Model file for the job. Use its own axes, mm. Face numbers are marked on the shaded views. A direction names the side the tool comes from. Give positions to 0.01 mm unless a question says otherwise; leave off trailing zeros. Loops run counter-clockwise (first coordinate to the right, second up) from the corner with the lowest first, then second, coordinate; pieces in that order, holes last. Notation, with made-up numbers: M -30,26 L -22,26 A9 cw -22,40 Z; hole C 32.25,44.25 d4. An arc over 180 degrees is marked long. Answer in a Markdown table with one row per item.
```python
from build123d import *

# Parameters (mm, degrees)
SKETCH1_W           = 25
SKETCH1_H           = 15.5
BOSS_EXTRUDE1_DEPTH = 15
SKETCH2_R           = 2.5
CUT_EXTRUDE1_DEPTH  = 10
SKETCH4_R           = 2.5
CUT_EXTRUDE3_DEPTH  = 4
SKETCH5_R           = 2.5
CUT_EXTRUDE4_DEPTH  = 4


with BuildPart() as part:
    # Sketch1 → Boss-Extrude1 (new body)
    with BuildSketch(Plane(origin=(0, 0, 0), x_dir=(1, 0, 0), z_dir=(0, 1, 0))):
        Rectangle(SKETCH1_W, SKETCH1_H)
    extrude(amount=BOSS_EXTRUDE1_DEPTH)

    # Sketch2 → Cut-Extrude1 (cut)
    with BuildSketch(Plane(origin=(0, 15, 0), x_dir=(1, 0, 0), z_dir=(0, 1, 0))):
        Circle(SKETCH2_R)
    extrude(amount=-CUT_EXTRUDE1_DEPTH, mode=Mode.SUBTRACT)

    # Sketch4 → Cut-Extrude3 (cut)
    with BuildSketch(Plane.XZ):
        with Locations((5, 0)):
            Circle(SKETCH4_R)
    extrude(amount=-CUT_EXTRUDE3_DEPTH, mode=Mode.SUBTRACT)

    # Sketch5 → Cut-Extrude4 (cut)
    with BuildSketch(Plane.XZ):
        with Locations((-5, 0)):
            Circle(SKETCH5_R)
    extrude(amount=-CUT_EXTRUDE4_DEPTH, mode=Mode.SUBTRACT)


solid = part.part
```
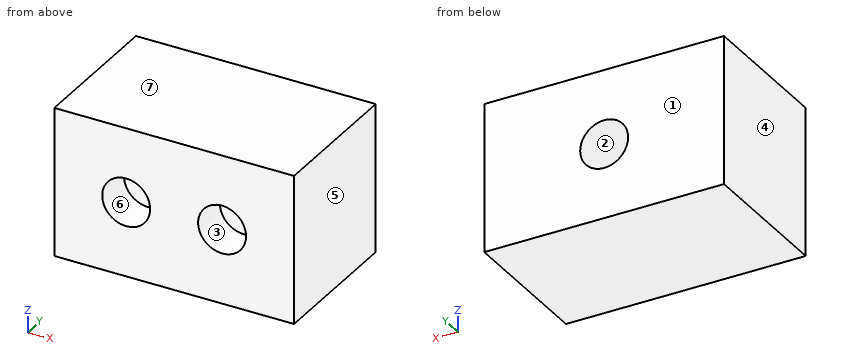
(1) Saw through at C-C, the plane y = 13.5. Give the cut face in (x, z).
Established:
| item | result |
|---|---|
| outline | M -12.5,-7.75 L 12.5,-7.75 L 12.5,7.75 L -12.5,7.75 Z; hole C 0,0 d5 |
(2) Saw through at B-B, the plane z = 0. Give the cut face in (x, y).
Established:
| item | result |
|---|---|
| outline | M -12.5,0 L -7.5,0 L -7.5,4 L -2.5,4 L -2.5,0 L 2.5,0 L 2.5,4 L 7.5,4 L 7.5,0 L 12.5,0 L 12.5,15 L 2.5,15 L 2.5,5 L -2.5,5 L -2.5,15 L -12.5,15 Z |
(3) Wall check: L1, parallel to Z at x = -5, y = 2.55; L2, parallel to X at y = 11.5, z = 0; L3, parallel to Y at x = 0, z = -0.5. Give the ranges that are in metal, low to high.
Established:
| item | result |
|---|---|
| L1 | z = -7.75 to -2.5, 2.5 to 7.75 |
| L2 | x = -12.5 to -2.5, 2.5 to 12.5 |
| L3 | y = 0 to 5 |
(4) Saw through at D-D, the plane x = -7. Give the cut face in (y, z).
Established:
| item | result |
|---|---|
| outline | M 0,-7.75 L 15,-7.75 L 15,7.75 L 0,7.75 L 0,1.5 L 4,1.5 L 4,-1.5 L 0,-1.5 Z |
(5) Which spindle directions (+Z, -Z, +X, -X, +Y, -Y) get a long thin tool onto all of the face, cutting with end or side? Do the marked faces 1, 2 and 3. Say none if no direction does.
Established:
| item | result |
|---|---|
| face 1 | +Z, -Z, +X, -X, +Y |
| face 2 | +Y |
| face 3 | -Y |
(6) Mould opens along X. For the marked faces 4, 5, 6 and 7 say: pulls with the +X half, pulls with the -X half, needs draft (parallel to the pull), parting line crosses it, or undercut.
Established:
| item | result |
|---|---|
| face 4 | pulls with the -X half |
| face 5 | pulls with the +X half |
| face 6 | undercut |
| face 7 | needs draft |
(7) Saw through at A-A, the plane x = 0. Give the cut face in (y, z).
Established:
| item | result |
|---|---|
| outline | M 0,-7.75 L 15,-7.75 L 15,-2.5 L 5,-2.5 L 5,2.5 L 15,2.5 L 15,7.75 L 0,7.75 Z |
